Read the model definition and answer for the solid it produces. Units are mm, in the model's axes. Face numbers are marked on the shaded views. Give positions to 0.01 mm unless a question says otherwise; leave off trailing zeros. Write each loop counter-clockwise with the first axis right and the second up, starting at its lowest first coordinate (ties: lowest second). Pieces come first, ordered by that corner, then holes. Notation, with made-up numbers: M 76,27.25 L 80,27.25 A18 cw 80,62.25 Z; hole C -26.75,59 d9. An arc over 180 degrees is marked long. Write each question's results on one line, items separated by ' | '. Start each with the question number.
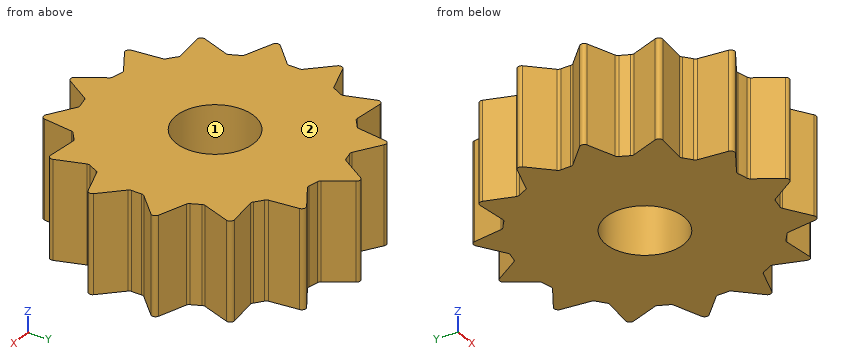
```python
from build123d import *

# Parameters (mm, degrees)
F0_R     = 1.000001
F1_DEPTH = 2.54
F2_R     = 0.1016


with BuildPart() as f1:
    # F0 (on Top) → F1 (new body)
    with BuildSketch(Plane.XY):
        with BuildLine():
            Line((0, 3.792523), (-0.508, 2.987927))
            ThreePointArc((-0.508, 2.987927), (-0.655986, 2.958962), (-0.802348, 2.922672))
            ThreePointArc((-0.802348, 2.922672), (-1.280873, 2.746841), (-1.723157, 2.493292))
            ThreePointArc((-1.723157, 2.493292), (-1.861136, 2.392059), (-1.993181, 2.2832))
            ThreePointArc((-1.993181, 2.2832), (-2.347676, 1.916818), (-2.635746, 1.496202))
            ThreePointArc((-2.635746, 1.496202), (-2.715992, 1.34505), (-2.78758, 1.189611))
            ThreePointArc((-2.78758, 1.189611), (-2.947537, 0.705549), (-3.024097, 0.201524))
            ThreePointArc((-3.024097, 0.201524), (-3.030651, 0.030517), (-3.027542, -0.140587))
            ThreePointArc((-3.027542, -0.140587), (-2.961147, -0.646051), (-2.81097, -1.133236))
            ThreePointArc((-2.81097, -1.133236), (-2.742527, -1.290085), (-2.66534, -1.442822))
            ThreePointArc((-2.66534, -1.442822), (-2.385799, -1.869154), (-2.038754, -2.2426))
            ThreePointArc((-2.038754, -2.2426), (-1.908928, -2.354096), (-1.773015, -2.458087))
            ThreePointArc((-1.773015, -2.458087), (-1.335927, -2.720491), (-0.86104, -2.905922))
            ThreePointArc((-0.86104, -2.905922), (-0.695652, -2.949889), (-0.528046, -2.98445))
            ThreePointArc((-0.528046, -2.98445), (-0.020345, -3.030736), (0.487931, -2.99127))
            ThreePointArc((0.487931, -2.99127), (0.655986, -2.958962), (0.821949, -2.91722))
            ThreePointArc((0.821949, -2.91722), (1.299283, -2.738181), (1.739855, -2.481668))
            ThreePointArc((1.739855, -2.481668), (1.877151, -2.379512), (2.008463, -2.269769))
            ThreePointArc((2.008463, -2.269769), (2.36049, -1.901016), (2.64573, -1.478475))
            ThreePointArc((2.64573, -1.478475), (2.72496, -1.326788), (2.795502, -1.170872))
            ThreePointArc((2.795502, -1.170872), (2.952207, -0.685747), (3.025382, -0.181219))
            ThreePointArc((3.025382, -0.181219), (3.030787, -0.010173), (3.02653, 0.160907))
            ThreePointArc((3.02653, 0.160907), (2.956744, 0.665914), (2.803299, 1.15208))
            ThreePointArc((2.803299, 1.15208), (2.733805, 1.308466), (2.655595, 1.460681))
            ThreePointArc((2.655595, 1.460681), (2.373198, 1.885127), (2.023654, 2.256236))
            ThreePointArc((2.023654, 2.256236), (1.893082, 2.366857), (1.756475, 2.469933))
            ThreePointArc((1.756475, 2.469933), (1.317635, 2.729398), (0.841513, 2.911637))
            ThreePointArc((0.841513, 2.911637), (0.675834, 2.954492), (0.508, 2.987927))
            Line((0.508, 2.987927), (0, 3.792523))
        make_face()
        Circle(F0_R, mode=Mode.SUBTRACT)
        with BuildLine():
            Line((1.64879, 3.415366), (0.841513, 2.911637))
            ThreePointArc((0.841513, 2.911637), (1.317635, 2.729398), (1.756475, 2.469933))
            Line((1.756475, 2.469933), (1.64879, 3.415366))
        make_face()
        with BuildLine():
            ThreePointArc((-1.723157, 2.493292), (-1.280873, 2.746841), (-0.802348, 2.922672))
            Line((-0.802348, 2.922672), (-1.60279, 3.437193))
            Line((-1.60279, 3.437193), (-1.723157, 2.493292))
        make_face()
        with BuildLine():
            ThreePointArc((-2.635746, 1.496202), (-2.347676, 1.916818), (-1.993181, 2.2832))
            Line((-1.993181, 2.2832), (-2.937707, 2.398564))
            Line((-2.937707, 2.398564), (-2.635746, 1.496202))
        make_face()
        with BuildLine():
            ThreePointArc((-3.024097, 0.201524), (-2.947537, 0.705549), (-2.78758, 1.189611))
            Line((-2.78758, 1.189611), (-3.688329, 0.882871))
            Line((-3.688329, 0.882871), (-3.024097, 0.201524))
        make_face()
        with BuildLine():
            ThreePointArc((-2.81097, -1.133236), (-2.961147, -0.646051), (-3.027542, -0.140587))
            Line((-3.027542, -0.140587), (-3.705359, -0.80842))
            Line((-3.705359, -0.80842), (-2.81097, -1.133236))
        make_face()
        with BuildLine():
            ThreePointArc((-2.038754, -2.2426), (-2.385799, -1.869154), (-2.66534, -1.442822))
            Line((-2.66534, -1.442822), (-2.985412, -2.338921))
            Line((-2.985412, -2.338921), (-2.038754, -2.2426))
        make_face()
        with BuildLine():
            ThreePointArc((-0.86104, -2.905922), (-1.335927, -2.720491), (-1.773015, -2.458087))
            Line((-1.773015, -2.458087), (-1.67168, -3.404221))
            Line((-1.67168, -3.404221), (-0.86104, -2.905922))
        make_face()
        with BuildLine():
            ThreePointArc((0.487931, -2.99127), (-0.020345, -3.030736), (-0.528046, -2.98445))
            Line((-0.528046, -2.98445), (-0.025458, -3.792438))
            Line((-0.025458, -3.792438), (0.487931, -2.99127))
        make_face()
        with BuildLine():
            Line((1.625826, -3.426357), (1.739855, -2.481668))
            ThreePointArc((1.739855, -2.481668), (1.299283, -2.738181), (0.821949, -2.91722))
            Line((0.821949, -2.91722), (1.625826, -3.426357))
        make_face()
        with BuildLine():
            Line((2.953742, -2.37879), (2.64573, -1.478475))
            ThreePointArc((2.64573, -1.478475), (2.36049, -1.901016), (2.008463, -2.269769))
            Line((2.008463, -2.269769), (2.953742, -2.37879))
        make_face()
        with BuildLine():
            Line((3.694172, -0.858093), (3.025382, -0.181219))
            ThreePointArc((3.025382, -0.181219), (2.952207, -0.685747), (2.795502, -1.170872))
            Line((2.795502, -1.170872), (3.694172, -0.858093))
        make_face()
        with BuildLine():
            Line((3.699849, 0.833275), (2.803299, 1.15208))
            ThreePointArc((2.803299, 1.15208), (2.956744, 0.665914), (3.02653, 0.160907))
            Line((3.02653, 0.160907), (3.699849, 0.833275))
        make_face()
        with BuildLine():
            Line((2.969644, 2.358908), (2.023654, 2.256236))
            ThreePointArc((2.023654, 2.256236), (2.373198, 1.885127), (2.655595, 1.460681))
            Line((2.655595, 1.460681), (2.969644, 2.358908))
        make_face()
    extrude(amount=F1_DEPTH)

    # F2
    f2_edges = [f1.edges().sort_by_distance(p)[0] for p in [
        (0, 3.792523, 1.27),
        (-1.60279, 3.437193, 1.27),
        (-2.937707, 2.398564, 1.27),
        (-3.688329, 0.882871, 1.27),
        (-3.705359, -0.80842, 1.27),
        (-2.985412, -2.338921, 1.27),
        (-1.67168, -3.404221, 1.27),
        (-0.025458, -3.792438, 1.27),
        (1.625826, -3.426357, 1.27),
        (2.953742, -2.37879, 1.27),
        (3.694172, -0.858093, 1.27),
        (3.699849, 0.833275, 1.27),
        (2.969644, 2.358908, 1.27),
        (1.64879, 3.415366, 1.27),
        (0.508, 2.987927, 1.27),
        (0.841513, 2.911637, 1.27),
        (1.756475, 2.469933, 1.27),
        (2.023654, 2.256236, 1.27),
        (2.655595, 1.460681, 1.27),
        (2.803299, 1.15208, 1.27),
        (3.02653, 0.160907, 1.27),
        (3.025382, -0.181219, 1.27),
        (2.795502, -1.170872, 1.27),
        (2.64573, -1.478475, 1.27),
        (2.008463, -2.269769, 1.27),
        (1.739855, -2.481668, 1.27),
        (0.821949, -2.91722, 1.27),
        (0.487931, -2.99127, 1.27),
        (-0.528046, -2.98445, 1.27),
        (-0.86104, -2.905922, 1.27),
        (-1.773015, -2.458087, 1.27),
        (-2.038754, -2.2426, 1.27),
        (-2.66534, -1.442822, 1.27),
        (-2.81097, -1.133236, 1.27),
        (-3.027542, -0.140587, 1.27),
        (-3.024097, 0.201524, 1.27),
        (-2.635746, 1.496202, 1.27),
        (-1.723157, 2.493292, 1.27),
        (-1.993181, 2.2832, 1.27),
        (-0.802348, 2.922672, 1.27),
        (-0.508, 2.987927, 1.27),
    ]]
    fillet(f2_edges, radius=F2_R)


solid = f1.part
```
Item 1: Section A-A, the plane y = 0 is taken. Determine the outline of the cut face in (x, z).
Item 2: Straight lines are drawn through the part: line 1 (Y direction, x = 0, z = 0.6); line 2 (X direction, y = -1.5, z = 1.4); line 3 (X direction, y = -0.25, z = 1.75). For each, find the intervals that lie inside material, in ascending order.
Item 3: Given P1, Ø1, axis at y = 0, z = 1, coming from the +X side, flat-ended and moving along its own axis, determine where the tip first touches the part or whether it passes through.
Item 4: Section B-B, the plane y = -2 is taken. Determine the outline of the cut face in (x, z).
Item 5: Determine the mould class of the marked faces 1 and 2 for opening direction X: +X half, -X half, draft (parallel to the pull), parting line (faces both ways), or undercut.
Worked out:
1) outline: M -3.03,0 L -1,0 L -1,2.54 L -3.03,2.54 Z; M 1,0 L 3.03,0 L 3.03,2.54 L 1,2.54 Z
2) line 1: y = -3.7 to -1, 1 to 3.7 | line 2: x = -2.69 to 2.66 | line 3: x = -3.14 to -0.97, 0.97 to 3.09
3) P1: stops at x = 3.37
4) outline: M -2.86,0 L 2.82,0 L 2.82,2.54 L -2.86,2.54 Z
5) face 1: undercut | face 2: draft
